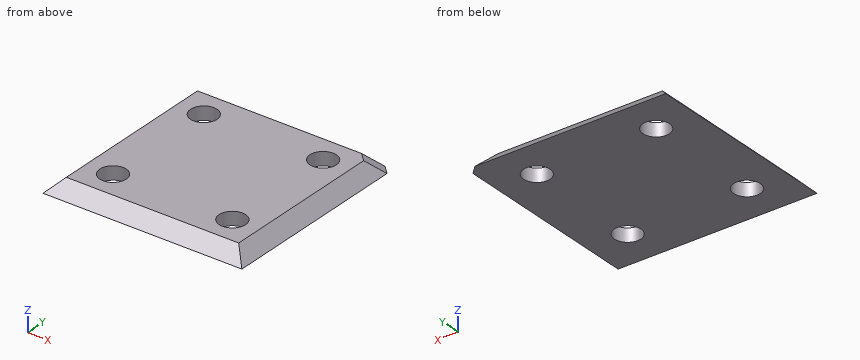
```python
from build123d import *

# Parameters (mm, degrees)
F0_W        = 76.2
F0_H        = 76.2
F1_DEPTH    = 5.08
F2_R        = 5.08
F3_DEPTH    = 25.4
F4_SIZE     = 5.07999
F5_T1_DEPTH = 21.9411964155


# Not quite as in the source:
# - a fillet or chamfer that OpenCascade refuses, or shapes differently, is made with other operations: its cross-section is extruded or revolved along the edge and cut away or added
# - a fillet or chamfer is up to 0.001 mm smaller than in the source, because OpenCascade refuses the exact size


with BuildPart() as f1:
    # F0 (on Top) → F1 (new body)
    with BuildSketch(Plane.XY):
        with Locations((38.1, 38.1)):
            Rectangle(F0_W, F0_H)
    extrude(amount=F1_DEPTH)

    # F2 (on face) → F3 (cut)
    with BuildSketch(Plane.XY.offset(5.08)):
        with Locations((15.24, 60.96)):
            Circle(F2_R)
        with Locations((60.96, 60.96)):
            Circle(F2_R)
        with Locations((15.24, 15.24)):
            Circle(F2_R)
        with Locations((60.96, 15.24)):
            Circle(F2_R)
    extrude(amount=-F3_DEPTH, mode=Mode.SUBTRACT)

    # F4 (size 5.08 in the source; OpenCascade refuses exactly that, so slightly less here)
    f4_edges = [f1.edges().sort_by_distance(p)[0] for p in [
        (38.1, 76.2, 5.08),
        (0, 38.1, 5.08),
        (76.2, 38.1, 5.08),
        (38.1, 0, 5.08),
    ]]
    chamfer(f4_edges, length=F4_SIZE)

    # F5: chamfer of 2.54 on 1 edges, made by hand

    # F5_s2 → F5_t1 (cut)
    with BuildSketch(Plane(origin=(54.5938794951, 54.5938794951, -54.5938794951), x_dir=(0.7071067812, -0.7071067812, 0), z_dir=(-0.5773502692, -0.5773502692, 0.5773502692))):
        Polygon((-2.1997045256, 60.9470476317), (2.1997045256, 60.9470476317), (0, 62.2170476317), align=None)
    extrude(amount=F5_T1_DEPTH, mode=Mode.SUBTRACT)


solid = f1.part
```
The listing builds one solid part. Answer for the finished solid, in the listing's coordinates (mm). Coordinates: 2 decimals unless noted, no trailing zeros. Loops run counter-clockwise (first coordinate to the right, second up) from the corner with the lowest first, then second, coordinate; pieces in that order, holes last. Notation, with made-up numbers: M -2,86 L 24,86 A13 ccw 24,110 Z; hole C -35.75,9.5 d3. An arc over 180 degrees is marked long. Answer as a JSON object with one key per item and string values. Group by question number.
Item 1: Each of these flat-tipped pins is pushed along its axis until it touches: P1, Ø1.5, axis at x = 10.5, z = 0.5, coming from the +Y side; P2, Ø8, axis at x = 15.24, y = 60.96, coming from the -Z side; P3, Ø1.5, axis at y = 42, z = 4.5, coming from the +X side; P4, Ø1.5, axis at y = 57.5, z = 2, coming from the +X side. Where does it stop, or does it pass through?
Item 2: Consider L1, parallel to Y at x = 61.5, z = 2.35; L2, parallel to Y at x = 15.24, z = 1.95; L3, parallel to X at y = 14, z = 3.8. Determine where each line is inside the solid, lowest interval first.
Item 3: Section C-C (z = 2.5) is taken. Write down the section's boundary in (x, y).
Item 4: Section A-A (x = 15.24) is taken. Give the number of separate pieces and of enclosed holes in the cut face, and give its area (3 significant figures).
Solved:
{
 "1": {"P1": "stops at y = 76.2", "P2": "passes through", "P3": "stops at x = 72.45", "P4": "stops at x = 74.95"},
 "2": {"L1": "y = 2.35 to 10.19, 20.29 to 55.91, 66.01 to 73.85", "L2": "y = 1.95 to 10.16, 20.32 to 55.88, 66.04 to 74.25", "L3": "x = 3.8 to 10.31, 20.17 to 56.03, 65.89 to 72.4"},
 "3": {"outline": "M 2.5,2.5 L 73.7,2.5 L 73.7,70.59 L 70.59,73.7 L 2.5,73.7 Z; hole C 15.24,15.24 d10.16; hole C 15.24,60.96 d10.16; hole C 60.96,15.24 d10.16; hole C 60.96,60.96 d10.16"},
 "4": {"separate pieces": "3", "enclosed holes": "0", "area": "258 mm2"}
}
